Answer from the drawing. Dimensions are ordinates in mm from the lowest x, y and z of the part. Coordinates: 2 decimals unless noted, no trailing zeros. Loops run counter-clockwise (first coordinate to the right, second up) from the corner with the lowest first, then second, coordinate; pieces in that order, holes last. Notation, with made-up numbers: (-3.5, -39.75) -> (53.5, -39.75) arc R18 ccw to (53.5, -23.75) -> close; hole circle Ø9 at (23.25, -8). An arc over 180 degrees is marked (long way). Answer as CSV lines item,"result".
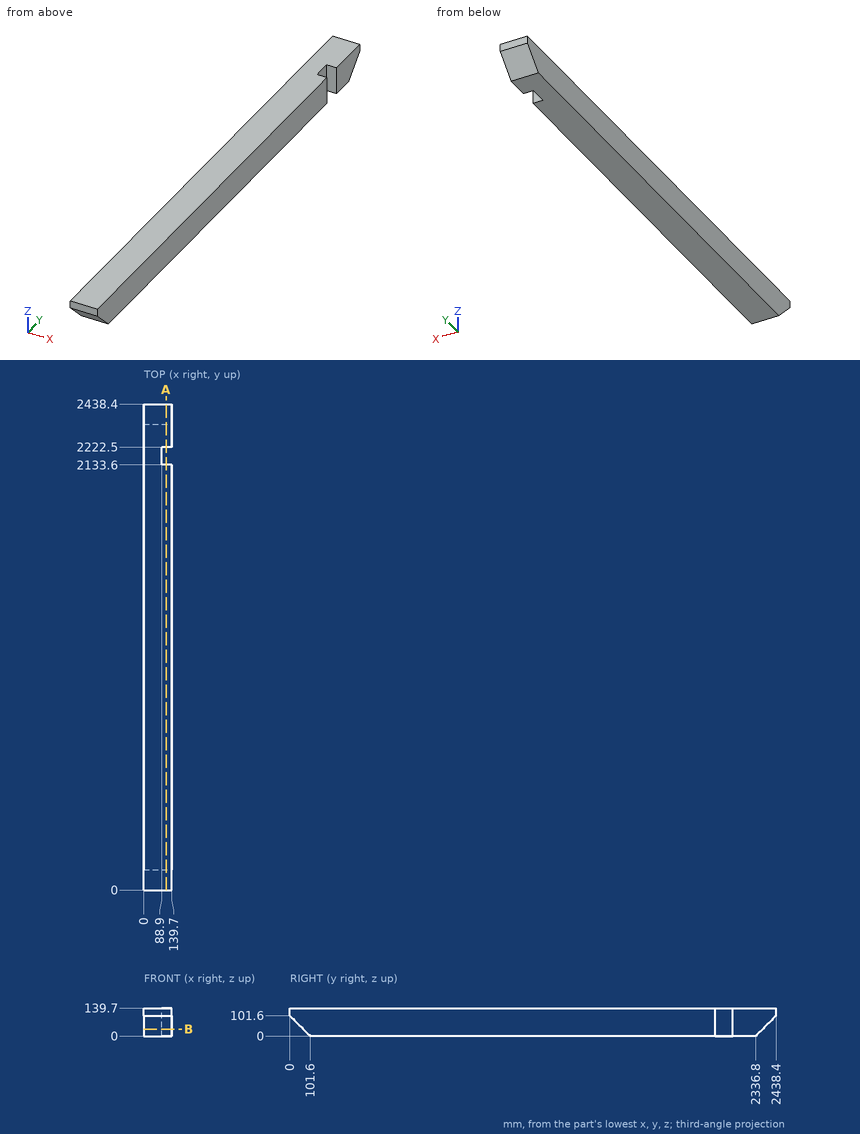
(1) A cutting plane is placed at A-A, the plane x = 111. Write down the section's boundary in (y, z).
Computed values:
outline,"(0, 101.6) -> (101.6, 0) -> (2133.6, 0) -> (2133.6, 139.7) -> (0, 139.7) -> close; (2222.5, 0) -> (2336.8, 0) -> (2438.4, 101.6) -> (2438.4, 139.7) -> (2222.5, 139.7) -> close"
(2) Flat-ended cylindrical pins translate along their axes: pin 1 Ø8 at (x, z) = (46, 118) entering from -Y; pin 2 Ø3 at (x, z) = (34, 48.5) entering from +Y; pin 3 Ø2 at (x, z) = (81.5, 47.5) entering from +Y; pin 4 Ø10 at (x, z) = (48, 58) entering from -Y. Find the tip coordinate at first contact, or state that the pin passes through.
Computed values:
pin 1,"y = 0"
pin 2,"y = 2386.8"
pin 3,"y = 2385.3"
pin 4,"y = 38.6"
(3) Consider line 1 along Y through (x, z) = (97.5, 55.5); line 2 along Y through (x, z) = (130, 48.5); line 3 along X through (y, z) = (2204.5, 126.5). Determine where each line is inside the solid, lowest interval first.
Computed values:
line 1,"46.1 to 2133.6, 2222.5 to 2392.3"
line 2,"53.1 to 2133.6, 2222.5 to 2385.3"
line 3,"0 to 88.9"
(4) A cutting plane is placed at B-B, the plane z = 34. Write down the section's boundary in (x, y).
Computed values:
outline,"(0, 67.6) -> (139.7, 67.6) -> (139.7, 2133.6) -> (88.9, 2133.6) -> (88.9, 2222.5) -> (139.7, 2222.5) -> (139.7, 2370.8) -> (0, 2370.8) -> close"
